from build123d import *

# Parameters (mm, degrees)
SKETCH1_W           = 35
SKETCH1_H           = 73
SKETCH1_W_2         = 30
SKETCH1_H_2         = 5
BOSS_EXTRUDE1_DEPTH = 5
SKETCH2_W           = 2
SKETCH2_H           = 2
BOSS_EXTRUDE2_DEPTH = 4.1
SKETCH4_W           = 13
SKETCH4_H           = 13
SKETCH4_R           = 2
BOSS_EXTRUDE3_DEPTH = 2
SKETCH7_W           = 30
SKETCH7_H           = 5
BOSS_EXTRUDE4_DEPTH = 20


with BuildPart() as part:
    # Sketch1 → Boss-Extrude1 (new body)
    with BuildSketch(Plane.XY):
        with Locations((0, 36.5)):
            Rectangle(SKETCH1_W, SKETCH1_H)
        with Locations((0, 64.5)):
            Rectangle(SKETCH1_W_2, SKETCH1_H_2, mode=Mode.SUBTRACT)
        with Locations((0, 57.5)):
            Rectangle(SKETCH1_W_2, SKETCH1_H_2, mode=Mode.SUBTRACT)
        with Locations((0, 50.5)):
            Rectangle(SKETCH1_W_2, SKETCH1_H_2, mode=Mode.SUBTRACT)
        with Locations((0, 43.5)):
            Rectangle(SKETCH1_W_2, SKETCH1_H_2, mode=Mode.SUBTRACT)
        with Locations((0, 36.5)):
            Rectangle(SKETCH1_W_2, SKETCH1_H_2, mode=Mode.SUBTRACT)
        with Locations((0, 29.5)):
            Rectangle(SKETCH1_W_2, SKETCH1_H_2, mode=Mode.SUBTRACT)
        with Locations((0, 22.5)):
            Rectangle(SKETCH1_W_2, SKETCH1_H_2, mode=Mode.SUBTRACT)
        with Locations((0, 15.5)):
            Rectangle(SKETCH1_W_2, SKETCH1_H_2, mode=Mode.SUBTRACT)
        with Locations((0, 8.5)):
            Rectangle(SKETCH1_W_2, SKETCH1_H_2, mode=Mode.SUBTRACT)
    extrude(amount=BOSS_EXTRUDE1_DEPTH)

    # Sketch2 → Boss-Extrude2 (add)
    with BuildSketch(Plane(origin=(0, 0, 0), x_dir=(-1, 0, 0), z_dir=(0, 0, -1))):
        with Locations((-3.05, 40)):
            Rectangle(SKETCH2_W, SKETCH2_H)
        with Locations((3.05, 40)):
            Rectangle(SKETCH2_W, SKETCH2_H)
        with Locations((-3.05, 54)):
            Rectangle(SKETCH2_W, SKETCH2_H)
        with Locations((3.05, 54)):
            Rectangle(SKETCH2_W, SKETCH2_H)
        with Locations((-3.05, 26)):
            Rectangle(SKETCH2_W, SKETCH2_H)
        with Locations((3.05, 26)):
            Rectangle(SKETCH2_W, SKETCH2_H)
        with Locations((-3.05, 12)):
            Rectangle(SKETCH2_W, SKETCH2_H)
        with Locations((3.05, 12)):
            Rectangle(SKETCH2_W, SKETCH2_H)
    extrude(amount=BOSS_EXTRUDE2_DEPTH)

    # Sketch4 → Boss-Extrude3 (add)
    # profile 1 of 4: a face of its own
    with BuildSketch(Plane.XY.offset(5)):
        with Locations((-22.75, 66.5)):
            Rectangle(SKETCH4_W, SKETCH4_H)
        with Locations((-22.75, 66.5)):
            Circle(SKETCH4_R, mode=Mode.SUBTRACT)
    # profile 2 of 4: a face of its own
    with BuildSketch(Plane.XY.offset(5)):
        with Locations((-22.75, 6.5)):
            Rectangle(SKETCH4_W, SKETCH4_H)
        with Locations(Location((-22.75, 6.5, 0), (0, 0, 180))):
            Circle(SKETCH4_R, mode=Mode.SUBTRACT)
    # profile 3 of 4: a face of its own
    with BuildSketch(Plane.XY.offset(5)):
        with Locations((22.75, 66.5)):
            Rectangle(SKETCH4_W, SKETCH4_H)
        with Locations(Location((22.75, 66.5, 0), (0, 0, 180))):
            Circle(SKETCH4_R, mode=Mode.SUBTRACT)
    # profile 4 of 4: a face of its own
    with BuildSketch(Plane.XY.offset(5)):
        with Locations((22.75, 6.5)):
            Rectangle(SKETCH4_W, SKETCH4_H)
        with Locations((22.75, 6.5)):
            Circle(SKETCH4_R, mode=Mode.SUBTRACT)
    extrude(amount=BOSS_EXTRUDE3_DEPTH)

    # Sketch7 → Boss-Extrude4 (add)
    with BuildSketch(Plane.XY):
        Polygon((-15, 69), (-15, 73), (-17.5, 73), (-17.5, 0), (-15, 0), (-15, 4), (15, 4), (15, 0), (17.5, 0), (17.5, 73), (15, 73), (15, 69), align=None)
        with Locations((0, 64.5)):
            Rectangle(SKETCH7_W, SKETCH7_H, mode=Mode.SUBTRACT)
        with Locations((0, 8.5)):
            Rectangle(SKETCH7_W, SKETCH7_H, mode=Mode.SUBTRACT)
        with Locations((0, 15.5)):
            Rectangle(SKETCH7_W, SKETCH7_H, mode=Mode.SUBTRACT)
        with Locations((0, 22.5)):
            Rectangle(SKETCH7_W, SKETCH7_H, mode=Mode.SUBTRACT)
        with Locations((0, 29.5)):
            Rectangle(SKETCH7_W, SKETCH7_H, mode=Mode.SUBTRACT)
        with Locations((0, 36.5)):
            Rectangle(SKETCH7_W, SKETCH7_H, mode=Mode.SUBTRACT)
        with Locations((0, 43.5)):
            Rectangle(SKETCH7_W, SKETCH7_H, mode=Mode.SUBTRACT)
        with Locations((0, 50.5)):
            Rectangle(SKETCH7_W, SKETCH7_H, mode=Mode.SUBTRACT)
        with Locations((0, 57.5)):
            Rectangle(SKETCH7_W, SKETCH7_H, mode=Mode.SUBTRACT)
    extrude(amount=BOSS_EXTRUDE4_DEPTH)


solid = part.part
Geometry: final body of the model. Coordinates: model frame, mm. A direction names the side the tool comes from. Coordinates: 2 decimals unless noted, no trailing zeros. Write each loop counter-clockwise with the first axis right and the second up, starting at its lowest first coordinate (ties: lowest second). Pieces come first, ordered by that corner, then holes. Notation, with made-up numbers: (16, 73) - (56, 73) arc R16 ccw to (56, 90) - close; hole circle Ø4 at (81, -13). An arc over 180 degrees is marked (long way). Return JSON: item names as keys, results as strings.
Item 1: Section query C-C (y = 40). Output: boundary loops of the cut face in (x, z).
Completed:
{"outline": "(-17.5, 0) - (-4.05, 0) - (-4.05, -4.1) - (-2.05, -4.1) - (-2.05, 0) - (2.05, 0) - (2.05, -4.1) - (4.05, -4.1) - (4.05, 0) - (17.5, 0) - (17.5, 20) - (-17.5, 20) - close"}
Item 2: Pull-direction query (Y, two-part tool) for faces 1 (the face through (0, 20, 10)), 2 (the face through (0, 6, 10)), 3 (the face through (-3, 12, -4.1)); classes: +Y half, -Y half, draft (parallel to the pull), parting line (faces both ways), or undercut.
Completed:
{"face 1": "undercut", "face 2": "undercut", "face 3": "draft"}
Item 3: Section query D-D (x = 23). Output: boundary loops of the cut face in (y, z).
Completed:
{"outline": "(0, 5) - (4.52, 5) - (4.52, 7) - (0, 7) - close; (8.48, 5) - (13, 5) - (13, 7) - (8.48, 7) - close; (60, 5) - (64.52, 5) - (64.52, 7) - (60, 7) - close; (68.48, 5) - (73, 5) - (73, 7) - (68.48, 7) - close"}
Item 4: Pin query (flat end, axial travel): pin 1 Ø10 at (x, z) = (5, 6.5) entering from +Y; pin 2 Ø3 at (x, y) = (-10.5, 45.5) entering from -Z; pin 3 Ø3 at (y, z) = (33.5, 15) entering from +X; pin 4 Ø7 at (x, z) = (6, 10.5) entering from +Y. Return the tip coordinate at first contact, or that it passes through.
Completed:
{"pin 1": "stops at y = 73", "pin 2": "stops at z = 0", "pin 3": "stops at x = 17.5", "pin 4": "stops at y = 69"}
Item 5: Reachability of faces 4 (the face through (-15, 36, 10)), 5 (the face through (-25, 7, 7)), 6 (the face through (25, 8, 5)), 7 (the face through (-4.05, 12, -2)), 8 (the face through (0, 71, 5)) from +Z, -Z, +X, -X, +Y, -Y: full face, straight path, thin tool, end or side. Return the list, or none.
Completed:
{"face 4": "+Z, -Z", "face 5": "+Z, -X, +Y, -Y", "face 6": "-Z, +X, +Y, -Y", "face 7": "-Z, -X, +Y, -Y", "face 8": "+Z, +Y"}
Item 6: Section query A-A (x = -19). Output: boundary loops of the cut face in (y, z), and give its area (3 significant figures).
Completed:
{"outline": "(0, 5) - (13, 5) - (13, 7) - (0, 7) - close; (60, 5) - (73, 5) - (73, 7) - (60, 7) - close", "area": "52.0 mm2"}
Item 7: Section query B-B (y = 51). Output: boundary loops of the cut face in (x, z), and give its area (3 significant figures).
Completed:
{"outline": "(-17.5, 0) - (-15, 0) - (-15, 20) - (-17.5, 20) - close; (15, 0) - (17.5, 0) - (17.5, 20) - (15, 20) - close", "area": "100 mm2"}
Item 8: Line query: L1, parallel to Y at x = 22.75, z = 6.5; L2, parallel to X at y = 65, z = 11.25; L3, parallel to Z at x = -5, y = 40.5. Output: solid intervals per line, ascending.
Completed:
{"L1": "y = 0 to 4.5, 8.5 to 13, 60 to 64.5, 68.5 to 73", "L2": "x = -17.5 to -15, 15 to 17.5", "L3": "z = 0 to 20"}
